from build123d import *

# Parameters (mm, degrees)
EXTRUDE_1_DEPTH          = 12.375
EXTRUDE_1_DEPTH_BACK     = 13
SKETCH_1_R               = 13
CUT_EXTRUDE_1_DEPTH      = 20
CUT_EXTRUDE_1_DEPTH_BACK = 10
SKETCH_2_R               = 10.5
SWEEP_1_PITCH            = 5.5
CUT_EXTRUDE_2_DEPTH      = 20
CUT_EXTRUDE_2_DEPTH_BACK = 20
SKETCH_6_R               = 45.002821291


with BuildPart() as part:
    # 草图1 → 凸台-拉伸1 (new, two sides: drawn at the far end of the back side and taken through both)
    with BuildSketch(Plane.XY.offset(-EXTRUDE_1_DEPTH_BACK)):
        Circle(SKETCH_1_R)
    extrude(amount=EXTRUDE_1_DEPTH + EXTRUDE_1_DEPTH_BACK)

    # 草图2 → 切除-拉伸1 (cut, two sides: drawn at the far end of the back side and taken through both)
    with BuildSketch(Plane.XY.offset(-CUT_EXTRUDE_1_DEPTH_BACK)):
        Circle(SKETCH_2_R)
    extrude(amount=CUT_EXTRUDE_1_DEPTH + CUT_EXTRUDE_1_DEPTH_BACK, mode=Mode.SUBTRACT)

    # 扫描1: the profile of 草图4 screwed along a right-hand helix of 2.25 turns, 14 arcs to a turn; built about Z, then put on its axis
    sweep_1_z = Axis((0, 0, 0), (0, 0, 1))
    sweep_1_corners = [(10.5, 0, 0), (10.5, 0.249236025, -2.989628974), (8.5, 0.207696687, -2.491357479), (8.5, 0.041539337, -0.498271496)]
    with BuildLine(mode=Mode.PRIVATE) as sweep_1_profile:
        Line(sweep_1_corners[0], sweep_1_corners[1])
        Line(sweep_1_corners[1], sweep_1_corners[2])
        Line(sweep_1_corners[2], sweep_1_corners[3])
        Line(sweep_1_corners[3], sweep_1_corners[0])
    sweep_1_cap = Face(sweep_1_profile.wire())
    sweep_1_turn_angles = [0, 12.857142857, 25.714285714, 38.571428571, 51.428571429, 64.285714286, 77.142857143, 90, 102.857142857, 115.714285714, 128.571428571, 141.428571429, 154.285714286, 167.142857143, 180, 192.857142857, 205.714285714, 218.571428571, 231.428571429, 244.285714286, 257.142857143, 270, 282.857142857, 295.714285714, 308.571428571, 321.428571429, 334.285714286, 347.142857143, 360]
    sweep_1_turn_weights = [1, 0.9749279121818236, 1, 0.9749279121818236, 1, 0.9749279121818236, 1, 0.9749279121818236, 1, 0.9749279121818236, 1, 0.9749279121818236, 1, 0.9749279121818236, 1, 0.9749279121818236, 1, 0.9749279121818236, 1, 0.9749279121818236, 1, 0.9749279121818236, 1, 0.9749279121818237, 1, 0.9749279121818236, 1, 0.9749279121818236, 1]
    sweep_1_turn_rails = [Edge.make_bspline([Vector(p[0], p[1], 0).rotate(sweep_1_z, sweep_1_turn_angles[k]) / sweep_1_turn_weights[k] + Vector(0, 0, p[2] + SWEEP_1_PITCH * sweep_1_turn_angles[k] / 360) for k in range(29)], [0, 0, 0, 1, 1, 2, 2, 3, 3, 4, 4, 5, 5, 6, 6, 7, 7, 8, 8, 9, 9, 10, 10, 11, 11, 12, 12, 13, 13, 14, 14, 14], 2, sweep_1_turn_weights) for p in sweep_1_corners]
    sweep_1_turn_sides = [Face.make_surface_from_curves(sweep_1_turn_rails[p[0]], sweep_1_turn_rails[p[1]]) for p in [(0, 1), (1, 2), (2, 3), (3, 0)]]
    sweep_1_last_angles = [720, 732.857142857, 745.714285714, 758.571428571, 771.428571429, 784.285714286, 797.142857143, 803.571428571, 810]
    sweep_1_last_weights = [1, 0.9749279121818237, 1, 0.9749279121818235, 1, 0.9749279121818237, 1, 0.9937122098932412, 1]
    sweep_1_last_rails = [Edge.make_bspline([Vector(p[0], p[1], 0).rotate(sweep_1_z, sweep_1_last_angles[k]) / sweep_1_last_weights[k] + Vector(0, 0, p[2] + SWEEP_1_PITCH * sweep_1_last_angles[k] / 360) for k in range(9)], [0, 0, 0, 1, 1, 2, 2, 3, 3, 4, 4, 4], 2, sweep_1_last_weights) for p in sweep_1_corners]
    sweep_1_last_sides = [Face.make_surface_from_curves(sweep_1_last_rails[p[0]], sweep_1_last_rails[p[1]]) for p in [(0, 1), (1, 2), (2, 3), (3, 0)]]
    sweep_1 = Plane(origin=(0, 0, 0), x_dir=(-0.7071067811865414, -0.7071067811865537, 0), z_dir=(0, 0, 1)) * Solid(Shell([*[p.moved(Location((0, 0, SWEEP_1_PITCH * i))) for i in range(2) for p in sweep_1_turn_sides], *sweep_1_last_sides, sweep_1_cap, sweep_1_cap.rotate(sweep_1_z, 810).moved(Location((0, 0, SWEEP_1_PITCH * 810 / 360)))]))
    add(sweep_1)

    # 草图6 → 切除-拉伸2 (cut, two sides: drawn at the far end of the back side and taken through both)
    with BuildSketch(Plane(origin=(0, 0, 0), x_dir=(-1, 0, 0), z_dir=(0, -1, 0)).offset(-CUT_EXTRUDE_2_DEPTH_BACK)):
        with Locations((-0.191121104, 48)):
            Circle(SKETCH_6_R)
    extrude(amount=CUT_EXTRUDE_2_DEPTH + CUT_EXTRUDE_2_DEPTH_BACK, mode=Mode.SUBTRACT)


solid = part.part
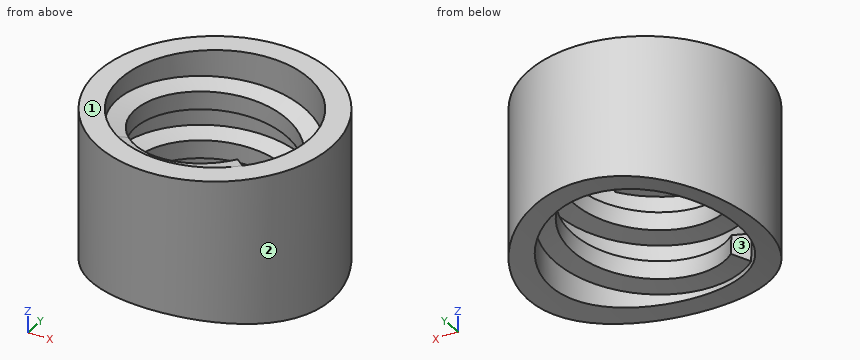
The model under review builds one solid part; all positions refer to its coordinate system, in mm. Face numbers are marked on the shaded views. Give positions to 0.01 mm unless a question says otherwise; leave off trailing zeros. One line per question, with ' | ' between items. Start each with the question number.
1) Clearance check with flat-ended pins moving along their axes: P1, Ø4, axis at y = -9.5, z = -3, coming from the +X side; P2, Ø12.5, axis at x = 0, y = 0, coming from the -Z side; P3, Ø6, axis at x = 5.5, z = 3.5, coming from the +Y side; P4, Ø10, axis at x = -5.5, z = 7, coming from the -Y side. State where each tip first meets the part, or that it passes through.
2) Wall thickness on L1, parallel to X at y = 0, z = 8.9; L2, parallel to X at y = -0.25, z = -2: over which ranges is each line inside the solid? List them lowest first. Write a range as from..to.
3) Mouldability with a two-part tool opening along Y and no side actions: class the marked faces 1, 2 and 3 as pulls with the +Y half, pulls with the -Y half, needs draft (parallel to the pull), parting line crosses it, or undercut.
4) Consider section A-A, the plane y = -6.5. State how many separate pieces and enclosed holes the cut face has, then the cut area to 3 significant figures.
Found:
1) P1: stops at x = 10.62 | P2: passes through | P3: stops at y = 12.76 | P4: stops at y = -12.99
2) L1: x = -13..-8.5, 10.5..13 | L2: x = -13..-10.5, 10.5..13
3) face 1: needs draft | face 2: parting line crosses it | face 3: undercut
4) separate pieces: 4 | enclosed holes: 0 | area: 131 mm²
